Input: part model. Units: mm. Frame: model coordinates. Face numbers are marked on the shaded views. Round coordinates to 2 decimals unless told otherwise and drop trailing zeros. Loops run counter-clockwise (first coordinate to the right, second up) from the corner with the lowest first, then second, coordinate; pieces in that order, holes last. Notation, with made-up numbers: (5.5, -20) - (38.5, -20) arc R24 ccw to (38.5, -7) - close; hole circle Ø1 at (60.25, 47.25). An arc over 180 degrees is marked (long way). Use CSV: the item, a comma, the result in double quotes. Start each with the question number.
1. Cut plane D-D (y = -27.5). Return loops of the section in (x, z), and give its area (3 significant figures).
2. Cut plane B-B (x = -39). Return loops of the section in (y, z).
3. Pull-direction query (X, two-part tool) for the marked faces 1 and 2; classes: +X half, -X half, draft (parallel to the pull), parting line (faces both ways), or undercut.
4. Cut plane C-C (z = 12). Give the number of separate pieces and of enclosed holes in the cut face, and give its area (3 significant figures).
5. Material intervals for probe 1 along Y at (x, z) = (-82.3, 16.25); probe 2 along Y at (x, z) = (-17.7, 16.5); probe 3 along X at (y, z) = (-9, 12.5), sorted ascending. Write a range as from..to.
6. Pin query (flat end, axial travel): P1, Ø1.8, axis at y = 11.5, z = 13, coming from the +X side; P2, Ø3, axis at x = 79, z = 13.5, coming from the +Y side; P3, Ø0.6, axis at x = -64, z = 16, coming from the -Y side. Return the tip coordinate at first contact, or that it passes through.
7. Cut plane A-A (x = -11). Return loops of the section in (y, z) (3 decimals), and give its area (3 significant figures).
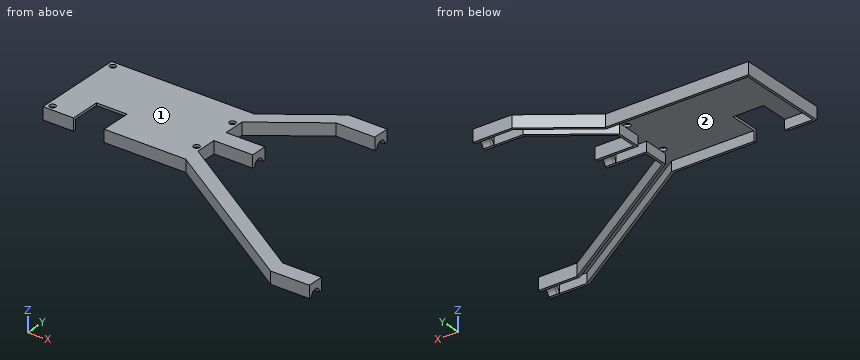
```python
from build123d import *

# Parameters (mm, degrees)
PAD001_DEPTH    = 6
THICKNESS001_T  = -1.2
SKETCH011_R     = 1.5
POCKET003_DEPTH = 1.2
SKETCH012_W     = 15
SKETCH012_H     = 15
POCKET004_DEPTH = 6.001
SKETCH013_R     = 2.6
POCKET005_DEPTH = 1.2
SKETCH014_R     = 2.6
POCKET006_DEPTH = 1.2
SKETCH015_R     = 2.6
POCKET007_DEPTH = 1.2
PAD008_DEPTH    = 4
PAD009_DEPTH    = 4
PAD010_DEPTH    = 4


with BuildPart() as part:
    # Sketch004 → Pad001 (new body)
    with BuildSketch(Plane.XY):
        Polygon((80, -74), (65, -74), (-15, -22.5), (-85, -22.5), (-85, 22.5), (-15, 22.5), (15, 44), (30, 44), (30, 36), (15, 36), (-15, 14.5), (-15, 4), (0, 4), (0, -4), (-15, -4), (-15, -14.5), (65, -66), (80, -66), align=None)
    extrude(amount=PAD001_DEPTH)

    # Thickness001
    thickness001_openings = [part.faces().sort_by_distance(p)[0] for p in [
        (-29.840547, -5.671982, 0),
    ]]
    offset(amount=THICKNESS001_T, openings=thickness001_openings, kind=Kind.INTERSECTION)

    # Sketch011 (on Face19 of Thickness001) → Pocket003 (cut)
    with BuildSketch(Plane.XY.offset(6)):
        with Locations((-82.3, 19.8)):
            Circle(SKETCH011_R)
        with Locations((-82.3, -19.8)):
            Circle(SKETCH011_R)
        with Locations((-17.7, 11.8)):
            Circle(SKETCH011_R)
        with Locations((-17.7, -11.8)):
            Circle(SKETCH011_R)
    extrude(amount=-POCKET003_DEPTH, mode=Mode.SUBTRACT)

    # Sketch012 (on Face5 of Pocket003) → Pocket004 (cut, through all)
    with BuildSketch(Plane.XY.offset(6)):
        with Locations((-62.5, -15)):
            Rectangle(SKETCH012_W, SKETCH012_H)
    extrude(amount=-POCKET004_DEPTH, mode=Mode.SUBTRACT)

    # Sketch013 (on Face16 of Pocket004) → Pocket005 (cut)
    with BuildSketch(Plane.YZ.offset(30)):
        with Locations((40, 0)):
            Circle(SKETCH013_R)
    extrude(amount=-POCKET005_DEPTH, mode=Mode.SUBTRACT)

    # Sketch014 (on Face11 of Pocket005) → Pocket006 (cut)
    with BuildSketch(Plane.YZ):
        Circle(SKETCH014_R)
    extrude(amount=-POCKET006_DEPTH, mode=Mode.SUBTRACT)

    # Sketch015 (on Face2 of Pocket006) → Pocket007 (cut)
    with BuildSketch(Plane.YZ.offset(80)):
        with Locations((-70, 0)):
            Circle(SKETCH015_R)
    extrude(amount=-POCKET007_DEPTH, mode=Mode.SUBTRACT)

    # Pocket007 Face2 → Pad008 (add)
    with BuildSketch(Plane(origin=(80, -70, 3.538728), x_dir=(0, -1, 0), z_dir=(1, 0, 0))):
        with BuildLine():
            Line((-2.6, 3.538728), (-4, 3.538728))
            Line((-4, 3.538728), (-4, -2.461272))
            Line((-4, -2.461272), (4, -2.461272))
            Line((4, -2.461272), (4, 3.538728))
            Line((4, 3.538728), (2.6, 3.538728))
            ThreePointArc((2.6, 3.538728), (0, 0.938728), (-2.6, 3.538728))
        make_face()
    extrude(amount=PAD008_DEPTH)

    # Pad008 Face12 → Pad009 (add)
    with BuildSketch(Plane(origin=(0, 0, 3.538728), x_dir=(0, -1, 0), z_dir=(1, 0, 0))):
        with BuildLine():
            Line((-2.6, 3.538728), (-4, 3.538728))
            Line((-4, 3.538728), (-4, -2.461272))
            Line((-4, -2.461272), (4, -2.461272))
            Line((4, -2.461272), (4, 3.538728))
            Line((4, 3.538728), (2.6, 3.538728))
            ThreePointArc((2.6, 3.538728), (0, 0.938728), (-2.6, 3.538728))
        make_face()
    extrude(amount=PAD009_DEPTH)

    # Pad009 Face19 → Pad010 (add)
    with BuildSketch(Plane(origin=(30, 40, 3.538728), x_dir=(0, -1, 0), z_dir=(1, 0, 0))):
        with BuildLine():
            Line((-2.6, 3.538728), (-4, 3.538728))
            Line((-4, 3.538728), (-4, -2.461272))
            Line((-4, -2.461272), (4, -2.461272))
            Line((4, -2.461272), (4, 3.538728))
            Line((4, 3.538728), (2.6, 3.538728))
            ThreePointArc((2.6, 3.538728), (0, 0.938728), (-2.6, 3.538728))
        make_face()
    extrude(amount=PAD010_DEPTH)


with BuildPart() as part_1:
    # Body001 placement: moved
    add(part.part.moved(Location((0, 0, 11))))


solid = part_1.part
```
Established:
1,outline,"(-7.23, 11) - (-5.02, 11) - (-5.02, 15.8) - (2.98, 15.8) - (2.98, 11) - (5.19, 11) - (5.19, 17) - (-7.23, 17) - close"
1,area,"36.2 mm2"
2,outline,"(-22.5, 11) - (-21.3, 11) - (-21.3, 15.8) - (21.3, 15.8) - (21.3, 11) - (22.5, 11) - (22.5, 17) - (-22.5, 17) - close"
3,face 1,"draft"
3,face 2,"undercut"
4,separate pieces,"4"
4,enclosed holes,"0"
4,area,"698 mm2"
5,probe 1,"y = -22.5..-21.3, -18.3..18.3, 21.3..22.5"
5,probe 2,"y = -22.5..-13.3, -10.3..10.3, 13.3..22.5"
5,probe 3,"x = -85..-83.8, -16.2..-15"
6,P1,"stops at x = -15"
6,P2,"stops at y = -66"
6,P3,"stops at y = -7.5"
7,outline,"(-25.075, 11) - (-23.648, 11) - (-23.648, 15.8) - (-18.502, 15.8) - (-18.502, 11) - (-17.075, 11) - (-17.075, 17) - (-25.075, 17) - close; (-4, 11) - (-2.8, 11) - (-2.8, 15.8) - (2.8, 15.8) - (2.8, 11) - (4, 11) - (4, 17) - (-4, 17) - close; (17.367, 11) - (18.843, 11) - (18.843, 15.8) - (23.89, 15.8) - (23.89, 11) - (25.367, 11) - (25.367, 17) - (17.367, 17) - close"
7,area,"68.2 mm2"
